Design review of the part built by this model. Coordinates are the model's own, in mm. A direction names the side the tool comes from. Coordinates: 2 decimals unless noted, no trailing zeros. Order: outer loops, then holes, each group sorted by start corner. A loop starts at its lowest first (then second) coordinate and runs counter-clockwise, first axis right, second up. Notation, with made-up numbers: (-36.5, 87.25) -> (10.5, 87.25) arc R21 cw to (10.5, 126.25) -> close; hole circle Ø5 at (64.5, 16.5). An arc over 180 degrees is marked (long way). Write item = value, one per line.
```python
from build123d import *

# Parameters (mm, degrees)
SKETCH_R  = 8
PAD_DEPTH = 200
FILLET_R  = 11


with BuildPart() as part:
    # Sketch → Pad (new body)
    with BuildSketch(Plane.XZ):
        with BuildLine():
            Line((-150, 15), (150, 15))
            Line((150, 15), (150, -15))
            Line((150, -15), (135, -15))
            ThreePointArc((105.267863, -15), (120.133931, -28), (135, -15))
            Line((105.267863, -15), (-105.267863, -15))
            ThreePointArc((-135, -15), (-120.133931, -28), (-105.267863, -15))
            Line((-135, -15), (-150, -15))
            Line((-150, -15), (-150, 15))
        make_face()
        with Locations((-120.133931, -13)):
            Circle(SKETCH_R, mode=Mode.SUBTRACT)
        with Locations((120.133931, -13)):
            Circle(SKETCH_R, mode=Mode.SUBTRACT)
    extrude(amount=PAD_DEPTH)

    # Fillet
    fillet_edges = [part.edges().sort_by_distance(p)[0] for p in [
        (-135, -100, -15),
        (-105.267863, -100, -15),
        (105.267863, -100, -15),
        (135, -100, -15),
    ]]
    fillet(fillet_edges, radius=FILLET_R)


solid = part.part
```
(1) We need section C-C (x = 12.5). Write out the cut boundary in (y, z), and give its area (3 significant figures).
Report:
outline = (-200, -15) -> (0, -15) -> (0, 15) -> (-200, 15) -> close
area = 6,000 mm²
(2) We need section B-B (y = -81.5). Write out the cut boundary in (x, z).
Report:
outline = (-150, -15) -> (-142.65, -15) arc R11 cw to (-133.12, -20.5) arc R15 ccw to (-107.14, -20.5) arc R11 cw to (-97.62, -15) -> (97.62, -15) arc R11 cw to (107.14, -20.5) arc R15 ccw to (133.12, -20.5) arc R11 cw to (142.65, -15) -> (150, -15) -> (150, 15) -> (-150, 15) -> close; hole circle Ø16 at (-120.13, -13); hole circle Ø16 at (120.13, -13)
(3) For L1, parallel to X at y = -97, z = -12; L2, parallel to X at y = -167, z = -9.5; L3, parallel to Z at x = -83, y = -185, list the stretches that pass through material, from the lowest coordinate up.
Report:
L1 = -150 to -128.07, -112.2 to 112.2, 128.07 to 150
L2 = -150 to -127.33, -112.94 to 112.94, 127.33 to 150
L3 = -15 to 15
(4) We need section A-A (z = -8). Write out the cut boundary in (x, y), and give its area (3 significant figures).
Report:
outline = (-150, -200) -> (-126.38, -200) -> (-126.38, 0) -> (-150, 0) -> close; (-113.89, -200) -> (113.89, -200) -> (113.89, 0) -> (-113.89, 0) -> close; (126.38, -200) -> (150, -200) -> (150, 0) -> (126.38, 0) -> close
area = 55,000 mm²
(5) The part is to be moulded in two halves that separate along X. For faces 1 (the cylindrical face through (-128.126, -98.6, -12.648)), 2 (the flat face through (150, -99, 0)), 3 (the cylindrical face through (-137.221, -101.4, -16.434)), 4 (the flat face through (-146, -99, -15)), say which applies: released by +X, released by -X, zero draft, split by the parting line, or undercut.
Report:
face_1 = undercut
face_2 = released by +X
face_3 = released by -X
face_4 = zero draft
(6) For faces 5 (the flat face through (-2, -99, 15)), 6 (the flat face through (1, -99, -15)), 7 (the flat face through (146, -99, -15)), list the 3-axis set-ups (+Z, -Z, +X, -X, +Y, -Y) from which the entire face can be reached by the end or side of a thin tool; tool diameter is ignored.
Report:
face_5 = +Z, +X, -X, +Y, -Y
face_6 = -Z, +Y, -Y
face_7 = -Z, +X, +Y, -Y
(7) Insertion check: pin 1 (1.5 mm diameter, centred on x = -76.5, y = -81.5, fed in from -Z); pin 2 (9.5 mm diameter, centred on x = -120.13, z = -13, fed in from +Y). Each pin has a flat end and moves straight along its axis. Give the tip position at first contact, or say it passes through.
Report:
pin_1 = -15
pin_2 = through
